from build123d import *

# Parameters (mm, degrees)
SKETCH1_R           = 26.5
SKETCH1_R_2         = 25
BOSS_EXTRUDE1_DEPTH = 55
SKETCH2_R           = 25
BOSS_EXTRUDE2_DEPTH = 2
BOSS_EXTRUDE3_START = 5
BOSS_EXTRUDE3_DEPTH = 5
SKETCH5_W           = 20
SKETCH5_H           = 10
CUT_EXTRUDE1_DEPTH  = 68
BOSS_EXTRUDE4_DEPTH = 2


with BuildPart() as part:
    # Sketch1 → Boss-Extrude1 (new body)
    with BuildSketch(Plane.XY):
        Circle(SKETCH1_R)
        Circle(SKETCH1_R_2, mode=Mode.SUBTRACT)
    extrude(amount=BOSS_EXTRUDE1_DEPTH)

    # Sketch2 → Boss-Extrude2 (add)
    with BuildSketch(Plane.XY.offset(55)):
        with BuildLine():
            Line((-26.330566677, 10.906477822), (-30.949964339, 12.819894984))
            ThreePointArc((-30.949964339, 12.819894984), (-33.5, 0), (-30.949964339, -12.819894984))
            Line((-30.949964339, -12.819894984), (-26.330566677, -10.906477822))
            ThreePointArc((-26.330566677, -10.906477822), (0, -28.5), (26.330566677, -10.906477822))
            Line((26.330566677, -10.906477822), (30.949964339, -12.819894984))
            ThreePointArc((30.949964339, -12.819894984), (33.5, 0), (30.949964339, 12.819894984))
            Line((30.949964339, 12.819894984), (26.330566677, 10.906477822))
            ThreePointArc((26.330566677, 10.906477822), (0, 28.5), (-26.330566677, 10.906477822))
        make_face()
        Circle(SKETCH2_R, mode=Mode.SUBTRACT)
    extrude(amount=BOSS_EXTRUDE2_DEPTH)

    # Sketch3 → Boss-Extrude3 (add)
    with BuildSketch(Plane(origin=(0, 0, 55), x_dir=(-1, 0, 0), z_dir=(0, 0, -1)).offset(BOSS_EXTRUDE3_START)):
        with BuildLine():
            ThreePointArc((-26.330566677, -10.906477822), (-28.5, 0), (-26.330566677, 10.906477822))
            Line((-26.330566677, 10.906477822), (-30.949964339, 12.819894984))
            ThreePointArc((-30.949964339, 12.819894984), (-33.5, 0), (-30.949964339, -12.819894984))
            Line((-30.949964339, -12.819894984), (-26.330566677, -10.906477822))
        make_face()
        with BuildLine():
            Line((30.949964339, 12.819894984), (26.330566677, 10.906477822))
            ThreePointArc((26.330566677, 10.906477822), (27.952380491, 5.560074177), (28.5, 0))
            ThreePointArc((28.5, 0), (27.952380491, -5.560074177), (26.330566677, -10.906477822))
            Line((26.330566677, -10.906477822), (30.949964339, -12.819894984))
            ThreePointArc((30.949964339, -12.819894984), (33.5, 0), (30.949964339, 12.819894984))
        make_face()
    extrude(amount=-BOSS_EXTRUDE3_DEPTH)

    # Sketch5 → Cut-Extrude1 (cut)
    with BuildSketch(Plane(origin=(0, 0, 20), x_dir=(-1, 0, 0), z_dir=(0, 0, -1))):
        with Locations((0, -25)):
            Rectangle(SKETCH5_W, SKETCH5_H)
    extrude(amount=CUT_EXTRUDE1_DEPTH, mode=Mode.SUBTRACT)

    # Sketch7 → Boss-Extrude4 (add)
    with BuildSketch(Plane(origin=(0, 0, 15), x_dir=(-1, 0, 0), z_dir=(0, 0, -1))):
        with BuildLine():
            ThreePointArc((-21.931712199, -12), (-23.475679338, -8.596073501), (-24.494897428, -5))
            Line((-24.494897428, -5), (-17.5, -5))
            ThreePointArc((-17.5, -5), (-14, -8.5), (-17.5, -12))
            Line((-17.5, -12), (-21.931712199, -12))
        make_face()
        with BuildLine():
            Line((21.931712199, -12), (17.5, -12))
            ThreePointArc((17.5, -12), (14, -8.5), (17.5, -5))
            Line((17.5, -5), (24.494897428, -5))
            ThreePointArc((24.494897428, -5), (23.475679338, -8.596073501), (21.931712199, -12))
        make_face()
    extrude(amount=-BOSS_EXTRUDE4_DEPTH)


solid = part.part
CAD build for the part. Positions are in the model's coordinates, mm. A direction names the side the tool comes from. Give positions to 0.01 mm unless a question says otherwise; leave off trailing zeros. Loops run counter-clockwise (first coordinate to the right, second up) from the corner with the lowest first, then second, coordinate; pieces in that order, holes last. Notation, with made-up numbers: M 1,-25.75 L 44,-25.75 A27 cw 44,8.25 Z; hole C -2,-3 d6. An arc over 180 degrees is marked long. One line per question, with ' | ' between items. Start each with the question number.
1. Flat gauge pins, fed straight in: pin 1 (1.3 mm diameter, centred on y = -23.5, z = 8.5, fed in from -X); pin 2 (5 mm diameter, centred on x = 1.5, z = 31.5, fed in from -Y); pin 3 (5.5 mm diameter, centred on x = 18, y = -7.5, fed in from -Z); pin 4 (5.5 mm diameter, centred on x = 29, y = 2.5, fed in from -Z). Where does each tip first touch, or does it go through?
2. Saw through at B-B on y = 14. Give the cut face in (x, z).
3. 3-axis set-ups, long thin cutter, end or side, ignore diameter. For faces 4 (the face through (14, -8.4, 16)), 5 (the face through (28.673, -11.877, 53.451)), 6 (the face through (19, -19, 55)): which of +Z, -Z, +X, -X, +Y, -Y reach the whole face in a straight line?
4. Two-plate mould, pull along Y, no slides. Class faces 1 (the face through (0.47, 28.496, 55.986)), 2 (the face through (-21, -5, 16)), 3 (the face through (10, -24, 10)): pulls with the +Y half, pulls with the -Y half, needs draft (parallel to the pull), parting line crosses it, or undercut.
5. Saw through at C-C on x = -2.5. Give the cut face in (y, z).
6. Probe L1, parallel to X at y = 0, z = 37.5; L2, parallel to Z at x = -27.5, y = -8.5. List the from-to ranges inside material, lowest first. Write a range as from..to.
7. Saw through at A-A on z = 51.5. Give the cut face in (x, y), plus the area to 3 significant figures.
8. Saw through at D-D on z = 45.5. Give the cut face in (x, y).
Result sheet:
1) pin 1: stops at x = -13.42 | pin 2: stops at y = -26.5 | pin 3: stops at z = 15 | pin 4: stops at z = 0
2) outline: M -24.82,55 L -22.5,55 L -22.5,0 L -20.71,0 L -20.71,57 L -24.82,57 Z; M 20.71,0 L 22.5,0 L 22.5,55 L 24.82,55 L 24.82,57 L 20.71,57 Z
3) face 4: +Z, -Z | face 5: +Z, -Z, -Y | face 6: -Z
4) face 1: pulls with the +Y half | face 2: undercut | face 3: needs draft
5) outline: M -28.39,55 L -26.38,55 L -26.38,20 L -24.87,20 L -24.87,57 L -28.39,57 Z; M 24.87,0 L 26.38,0 L 26.38,55 L 28.39,55 L 28.39,57 L 24.87,57 Z
6) L1: x = -26.5..-25, 25..26.5 | L2: z = 50..57
7) outline: M -30.95,-12.82 L -26.33,-10.91 A28.5 cw -26.33,10.91 L -30.95,12.82 A33.5 ccw Z; C 0,0 d53; M 26.33,-10.91 L 30.95,-12.82 A33.5 ccw 30.95,12.82 L 26.33,10.91 A28.5 cw Z; hole C 0,0 d50 | area: 486 mm^2
8) outline: C 0,0 d53; hole C 0,0 d50
